from build123d import *

# Parameters (mm, degrees)
F1_DEPTH = 6.35
F2_R     = 6.35
F3_D     = 10.16
F4_D     = 5.08


with BuildPart() as f1:
    # F0 (on Top) → F1 (new body)
    with BuildSketch(Plane.XY):
        Polygon((99.21875, -63.5), (99.21875, 127), (73.81875, 127), (-99.21875, 12.7), (-99.21875, -15.2791400352), (-99.21875, -20.9632049465), (-99.21875, -44.45), (73.81875, -63.5), align=None)
        Polygon((61.11875, -38.6150398089), (-80.955676291, -22.9738185659), (61.11875, 16.1292345417), align=None, mode=Mode.SUBTRACT)
        Polygon((61.11875, 35.8875947884), (-80.955676291, -3.2154583192), (61.11875, 90.6318691391), align=None, mode=Mode.SUBTRACT)
    extrude(amount=F1_DEPTH)

    # F2
    f2_edges = [f1.edges().sort_by_distance(p)[0] for p in [
        (99.21875, -63.5, 3.175),
        (99.21875, 127, 3.175),
        (-80.955676, -3.215458, 3.175),
        (-80.955676, -22.973819, 3.175),
        (61.11875, 90.631869, 3.175),
        (61.11875, 16.129235, 3.175),
        (61.11875, -38.61504, 3.175),
        (61.11875, 35.887595, 3.175),
        (-99.21875, -44.45, 3.175),
        (73.81875, -63.5, 3.175),
        (73.81875, 127, 3.175),
        (-99.21875, 12.7, 3.175),
    ]]
    fillet(f2_edges, radius=F2_R)

    # F3 (through all)
    with Locations(Plane(origin=(0, 0, 0), x_dir=(1, 0, 0), z_dir=(0, 0, -1))):
        with Locations((80.16875, -107.95), (80.16875, 44.45)):
            Hole(F3_D / 2)

    # F4 (through all)
    with Locations(Plane(origin=(0, 0, 0), x_dir=(1, 0, 0), z_dir=(0, 0, -1))):
        with Locations((91.1368808609, -118.9181308609), (69.2006191391, -96.9818691391), (91.3940701513, 55.6753201513), (68.9434298487, 33.2246798487), (-61.11875, 31.75), (-92.86875, 0), (-61.11875, 0), (-92.86875, 31.75)):
            Hole(F4_D / 2)


solid = f1.part
CAD build for the part. Positions are in the model's coordinates, mm. A direction names the side the tool comes from. Round coordinates to 2 decimals unless told otherwise and drop trailing zeros. Write each loop counter-clockwise with the first axis right and the second up, starting at its lowest first coordinate (ties: lowest second). Pieces come first, ordered by that corner, then holes. Notation, with made-up numbers: M -27.75,-19.75 L 16.25,-19.75 A24 ccw 16.25,11.25 Z; hole C -18.5,85 d3. An arc over 180 degrees is marked long. Use a Markdown table: item, result. Add a question column.
1. Slice it at B-B on x = -18.5. Give the cut face in (y, z).
2. Flat gauge pins, fed straight in: P1, Ø1.9, axis at y = 63, z = 4, coming from the -X side; P2, Ø6, axis at x = -61.12, y = 0, coming from the +Z side. Where does each tip first touch, or does it go through?
3. Drill centre lines: probe 1 along Y at (x, z) = (51, 0.5); probe 2 along Y at (x, z) = (9, 4.5); probe 3 along X at (y, z) = (-39, 5.25). Where is each one in solid material? Low to high.
4. Slice it at A-A on y = 107.95. Give the cut face in (x, z), then the cut area to 3 significant figures.
5. Slice it at C-C on z = 5. Give the number of separate pieces and of enclosed holes in the cut face, then the cut area to 3 significant figures.
6. 3-axis set-ups, long thin cutter, end or side, ignore diameter. For faces 4 (the face through (59.85, 36.92, 3.22)), 5 (the face through (21, 12, 0)): which of +Z, -Z, +X, -X, +Y, -Y reach the whole face in a straight line?
7. Slice it at D-D on y = 0. Give the cut face in (x, z).
8. Pull direction Y, two halves, no side cores. Call faces 1 (the face through (97.4, 125.1, 3.2)), 2 (the face through (99.219, 31, 3)), 3 (the face through (-53.622, -20.674, 3.219)): released by +Y, released by -Y, zero draft, split by the parting line, or undercut.
Reply:
| question | item | result |
|---|---|---|
| 1 | outline | M -53.34,0 L -29.85,0 L -29.85,6.35 L -53.34,6.35 Z; M -5.78,0 L 13.97,0 L 13.97,6.35 L -5.78,6.35 Z; M 38.04,0 L 66.02,0 L 66.02,6.35 L 38.04,6.35 Z |
| 2 | P1 | stops at x = -24.51 |
| 2 | P2 | stops at z = 6.35 |
| 3 | probe 1 | y = -60.99 to -37.5, 13.34 to 33.1, 83.95 to 111.93 |
| 3 | probe 2 | y = -56.36 to -32.88, 1.78 to 21.54, 56.2 to 84.18 |
| 3 | probe 3 | x = -99.21 to 99.22 |
| 4 | outline | M 44.98,0 L 75.09,0 L 75.09,6.35 L 44.98,6.35 Z; M 85.25,0 L 99.22,0 L 99.22,6.35 L 85.25,6.35 Z |
| 4 | area | 280 mm^2 |
| 5 | separate pieces | 1 |
| 5 | enclosed holes | 12 |
| 5 | area | 18,600 mm^2 |
| 6 | face 4 | +Z, -Z |
| 6 | face 5 | -Z, +X, -X, +Y, -Y |
| 7 | outline | M -99.22,0 L -95.41,0 L -95.41,6.35 L -99.22,6.35 Z; M -90.33,0 L -63.66,0 L -63.66,6.35 L -90.33,6.35 Z; M -58.58,0 L 2.52,0 L 2.52,6.35 L -58.58,6.35 Z; M 61.12,0 L 99.22,0 L 99.22,6.35 L 61.12,6.35 Z |
| 8 | face 1 | released by +Y |
| 8 | face 2 | zero draft |
| 8 | face 3 | undercut |
